Answer from the drawing. Dimensions are ordinates in mm from the lowest x, y and z of the part. Give positions to 0.01 mm unless a question says otherwise; leave off trailing zeros. Write each loop counter-clockwise with the first axis right and the second up, starting at its lowest first coordinate (ties: lowest second). Pieces come first, ordered by that corner, then holes. Notation, with made-up numbers: (23.5, 68.5) - (50.5, 68.5) arc R11 ccw to (50.5, 82.5) - close; hole circle Ø4 at (-28, 28). An arc over 180 degrees is marked (long way). Write item = value, one per line.
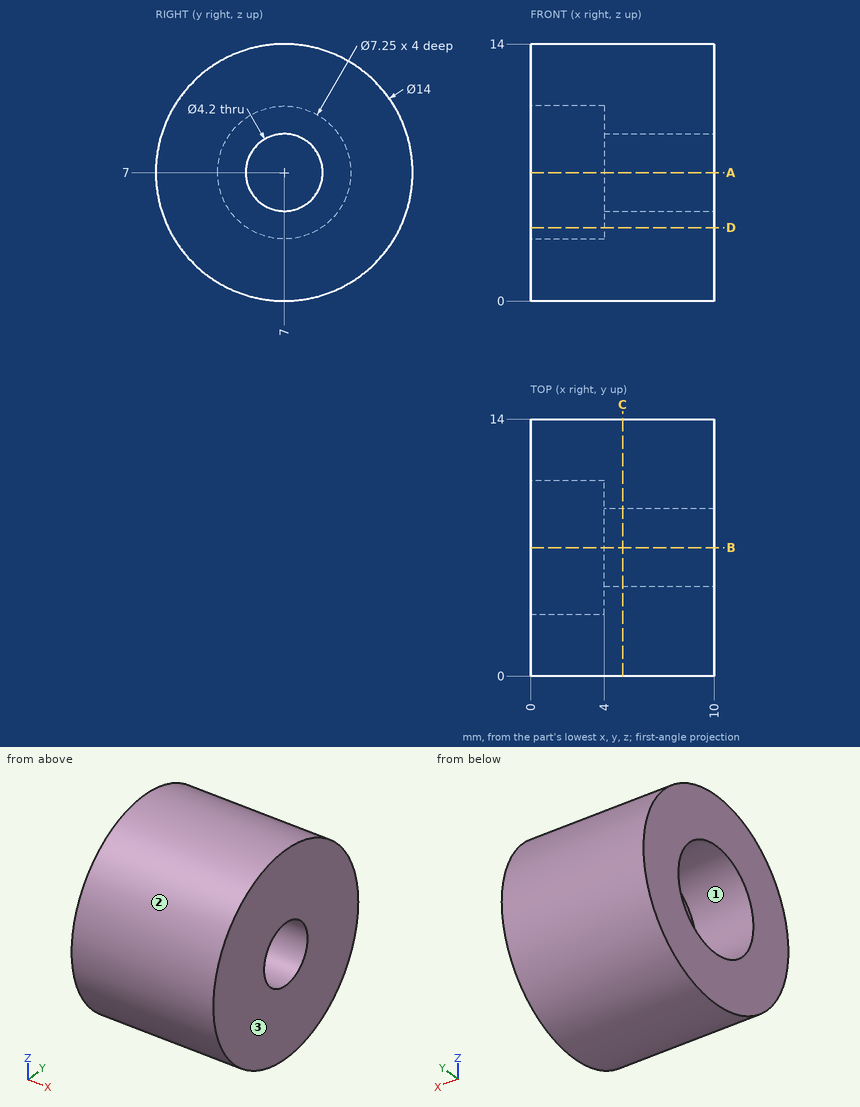
1. Find section A-A, the plane z = 7. Give the vertices of the cut face in (x, y) (3 decimals), then the cut area to 3 significant figures.
Solution:
outline = (0, 0) - (10, 0) - (10, 4.9) - (4, 4.9) - (4, 3.375) - (0, 3.375) - close; (0, 10.625) - (4, 10.625) - (4, 9.1) - (10, 9.1) - (10, 14) - (0, 14) - close
area = 85.8 mm^2
2. Find section C-C, the plane x = 5. Give the vertices of the cut face in (y, z).
Solution:
outline = circle Ø14 at (7, 7); hole circle Ø4.2 at (7, 7)
3. For a pull along Z with two mould halves and no side action, classify the marked faces 1, 2 and 3 as pulls with the +Z half, pulls with the -Z half, needs draft (parallel to the pull), parting line crosses it, or undercut.
Solution:
face_1 = undercut
face_2 = parting line crosses it
face_3 = needs draft
4. Given pin 1 (5 mm diameter, centred on x = 8.5, y = 12.5, fed in from -Z); pin 2 (1.5 mm diameter, centred on x = 3.5, z = 1.5, fed in from -Y); pin 3 (4 mm diameter, centred on y = 7, z = 7, fed in from +X), each flat-ended and moving along its own axis, determine where each tip first touches the part or whether it passes through.
Solution:
pin_1 = 0.68
pin_2 = 1.86
pin_3 = through
5. Straight lines are drawn through the part: line 1 (Z direction, x = 3.05, y = 7) (3 decimals); line 2 (Z direction, x = 8.25, y = 7); line 3 (Y direction, x = 2.75, z = 8). For each, find the intervals that lie inside material, in ascending order.
Solution:
line_1 = 0 to 3.375, 10.625 to 14
line_2 = 0 to 4.9, 9.1 to 14
line_3 = 0.07 to 3.52, 10.48 to 13.93
6. Find section D-D, the plane z = 4. Give the vertices of the cut face in (x, y).
Solution:
outline = (0, 0.68) - (10, 0.68) - (10, 13.32) - (0, 13.32) - (0, 9.03) - (4, 9.03) - (4, 4.97) - (0, 4.97) - close
